Work out the finished part from the listing and answer in its coordinate system (mm). A direction names the side the tool comes from. Round coordinates to 2 decimals unless told otherwise and drop trailing zeros. Write each loop counter-clockwise with the first axis right and the second up, starting at its lowest first coordinate (ties: lowest second). Pieces come first, ordered by that corner, then holes.
1. A tool of negligible diameter and unlimited length cuts with its end or side. For faces 1 (the face through (0.57, 56.874, 27.999)), 2 (the face through (93.1, 4.86, 39.77)), from which of +Z, -Z, +X, -X, +Y, -Y can it reach the whole face along a straight path? Write none if from no direction.
2. Find section B-B (y = 9.5). Write down the section's boundary in (x, z).
3. Straight lines are drawn through the part: probe 1 along X at (y, z) = (17, 37); probe 2 along Z at (x, y) = (27.5, 10); probe 3 along Y at (x, z) = (78.5, 29). For each, find the intervals that lie inside material, in ascending order.
4. Flat-ended cylindrical pins translate along their axes: pin 1 Ø6 at (x, z) = (68, 17) entering from +Y; pin 2 Ø3 at (x, y) = (26.5, 48.5) entering from +Z; pin 3 Ø6 at (x, y) = (14.5, 30.5) entering from +Z. Find the tip coordinate at first contact, or state that the pin passes through.
5. Determine the mould class of faces 3 (the face through (48.34, 57.71, 27.41)), 4 (the face through (97.43, 23.94, 58.4)), 5 (the face through (48, 4, 40)) for opening direction Y: pulls with the +Y half, pulls with the -Y half, needs draft (parallel to the pull), parting line crosses it, or undercut.
6. Find section A-A (x = 55). Write down the section's boundary in (y, z), and give its area (3 significant figures).
```python
from build123d import *

# Parameters (mm, degrees)
F1_DEPTH    = 98
F3_DEPTH    = 39
F4_T1_DEPTH = 123
F4_T3_DEPTH = 115.9227425884
F5_R        = 2


# Not quite as in the source:
# - a fillet or chamfer that OpenCascade refuses, or shapes differently, is made with other operations: its cross-section is extruded or revolved along the edge and cut away or added


with BuildPart() as f1:
    # F0 (on Right) → F1 (new body)
    with BuildSketch(Plane.YZ):
        Polygon((0, 59), (0, 0), (67, 0), (47, 59), align=None)
    extrude(amount=F1_DEPTH)

    # F2 (on face) → F3 (cut)
    with BuildSketch(Plane.XY.offset(59)):
        with BuildLine():
            Line((91, 43), (7, 43))
            ThreePointArc((7, 43), (4.8786796564, 42.1213203436), (4, 40))
            Line((4, 40), (4, 7))
            ThreePointArc((4, 7), (4.8786796564, 4.8786796564), (7, 4))
            Line((7, 4), (91, 4))
            ThreePointArc((91, 4), (93.1213203436, 4.8786796564), (94, 7))
            Line((94, 7), (94, 40))
            ThreePointArc((94, 40), (93.1213203436, 42.1213203436), (91, 43))
        make_face()
    extrude(amount=-F3_DEPTH, mode=Mode.SUBTRACT)

    # F4: fillet of radius 5 on 2 edges, made by hand

    # F4_s2 → F4_t1 (cut)
    with BuildSketch(Plane.YZ.offset(-12.5)):
        with BuildLine():
            ThreePointArc((0, 54), (1.4644660941, 57.5355339059), (5, 59))
            Line((5, 59), (0, 59))
            Line((0, 59), (0, 54))
        make_face()
    extrude(amount=F4_T1_DEPTH, mode=Mode.SUBTRACT)

    # F4_s4 → F4_t3 (cut)
    with BuildSketch(Plane.YZ.offset(-8.9613712942)):
        with BuildLine():
            ThreePointArc((43.4154514823, 59), (46.3286986372, 58.063617971), (48.1507808794, 55.6051964058))
            Line((48.1507808794, 55.6051964058), (47, 59))
            Line((47, 59), (43.4154514823, 59))
        make_face()
    extrude(amount=F4_T3_DEPTH, mode=Mode.SUBTRACT)

    # F5
    f5_edges = [f1.edges().sort_by_distance(p)[0] for p in [
        (0, 24.207726, 59),
        (98, 24.207726, 59),
        (0, 0, 27),
        (98, 0, 27),
        (0, 1.464466, 57.535534),
        (0, 46.328699, 58.063618),
        (0, 57.57539, 27.802598),
        (98, 1.464466, 57.535534),
        (98, 46.328699, 58.063618),
        (98, 57.57539, 27.802598),
    ]]
    fillet(f5_edges, radius=F5_R)


solid = f1.part
```
Worked answers:
1. face 1: +Z, -X, +Y
1. face 2: +Z
2. outline: (0, 0) - (98, 0) - (98, 57) arc R2 ccw to (96, 59) - (94, 59) - (94, 20) - (4, 20) - (4, 59) - (2, 59) arc R2 ccw to (0, 57) - close
3. probe 1: x = 0 to 4, 94 to 98
3. probe 2: z = 0 to 20
3. probe 3: y = 0 to 4, 43 to 57.17
4. pin 1: stops at y = 62.25
4. pin 2: stops at z = 57.49
4. pin 3: stops at z = 20
5. face 3: pulls with the +Y half
5. face 4: needs draft
5. face 5: undercut
6. outline: (0, 0) - (67, 0) - (48.15, 55.61) arc R5 ccw to (43.42, 59) - (43, 59) - (43, 20) - (4, 20) - (4, 58.9) arc R5 ccw to (0, 54) - close
6. area: 1,830 mm2
